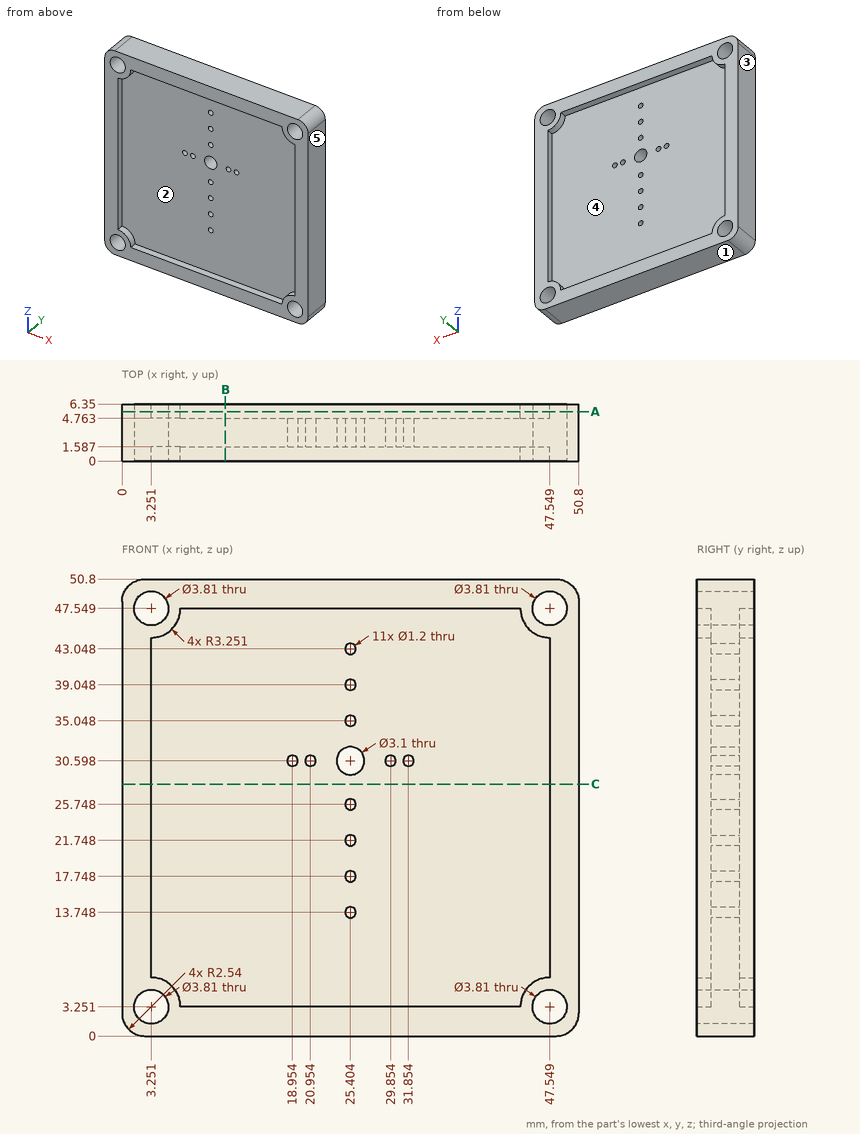
Input: dimensioned drawing with shaded views. Units: mm. Origin: part minimum x, y, z. A direction names the side the tool comes from. Give positions to 0.01 mm unless a question says otherwise; leave off trailing zeros. Loops run counter-clockwise (first coordinate to the right, second up) from the corner with the lowest first, then second, coordinate; pieces in that order, holes last. Notation, with made-up numbers: (26, 34) -> (33, 34) arc R30 ccw to (33, 60) -> close; hole circle Ø1 at (47.25, -37). An arc over 180 degrees is marked (long way). Use a Markdown table: item, result. Add a question column.
1) Section query A-A, the plane y = 5.5. Return the cut outline in (x, z) (1 decimal).
2) First-contact query: pin 1 (13.5 mm diameter, centred on x = 30.5, z = 17.5, fed in from +Y); pin 2 (1 mm diameter, centred on x = 39.5, z = 33.5, fed in from -Y). Flat tips, straight axial feed; report the tip coordinate or a pass-through.
3) Reachability of the marked faces 4 and 5 from +Z, -Z, +X, -X, +Y, -Y: full face, straight path, thin tool, end or side. Return the list, or none.
4) Section query B-B, the plane x = 11.5. Return the cut outline in (y, z).
5) Line query: line 1 along Z through (x, y) = (31.5, 5.75); line 2 along X through (y, z) = (4.5, 47) (1 decimal). Output: solid intervals per line, ascending. Write a range as [from, to].
6) Pull-direction query (Z, two-part tool) for the marked faces 1, 2 and 3; classes: +Z half, -Z half, draft (parallel to the pull), parting line (faces both ways), or undercut.
7) Section query C-C, the plane z = 28. Return the cut outline in (x, y), then the cut area to 3 significant figures.
Numbers:
| question | item | result |
|---|---|---|
| 1 | outline | (0, 2.5) arc R2.5 ccw to (2.5, 0) -> (48.3, 0) arc R2.5 ccw to (50.8, 2.5) -> (50.8, 48.3) arc R2.5 ccw to (48.3, 50.8) -> (2.5, 50.8) arc R2.5 ccw to (0, 48.3) -> close; hole circle Ø3.8 at (3.3, 3.3); hole circle Ø3.8 at (3.3, 47.5); hole (3.3, 6.5) arc R3.3 cw to (6.5, 3.3) -> (44.3, 3.3) arc R3.3 cw to (47.5, 6.5) -> (47.5, 44.3) arc R3.3 cw to (44.3, 47.5) -> (6.5, 47.5) arc R3.3 cw to (3.3, 44.3) -> close; hole circle Ø3.8 at (47.5, 3.3); hole circle Ø3.8 at (47.5, 47.5) |
| 2 | pin 1 | stops at y = 4.76 |
| 2 | pin 2 | stops at y = 1.59 |
| 3 | face 4 | +Y |
| 3 | face 5 | +Z, -Z, +X, +Y, -Y |
| 4 | outline | (0, 0) -> (6.35, 0) -> (6.35, 3.25) -> (4.76, 3.25) -> (4.76, 47.55) -> (6.35, 47.55) -> (6.35, 50.8) -> (0, 50.8) -> (0, 47.55) -> (1.59, 47.55) -> (1.59, 3.25) -> (0, 3.25) -> close |
| 5 | line 1 | z = [0, 3.25], [47.55, 50.8] |
| 5 | line 2 | x = [0, 1.4], [5.1, 45.7], [49.4, 50.8] |
| 6 | face 1 | -Z half |
| 6 | face 2 | undercut |
| 6 | face 3 | draft |
| 7 | outline | (0, 0) -> (3.25, 0) -> (3.25, 1.59) -> (47.55, 1.59) -> (47.55, 0) -> (50.8, 0) -> (50.8, 6.35) -> (47.55, 6.35) -> (47.55, 4.76) -> (3.25, 4.76) -> (3.25, 6.35) -> (0, 6.35) -> close |
| 7 | area | 182 mm2 |
